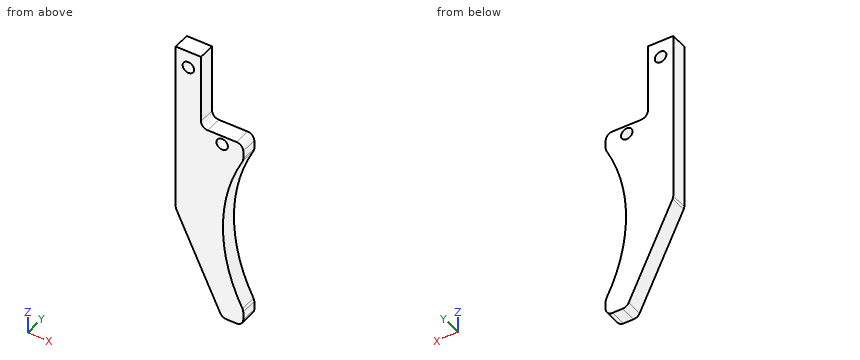
from build123d import *

# Parameters (mm, degrees)
BOSS_EXTRUDE1_DEPTH     = 6.35
CUT_EXTRUDE2_DEPTH      = 105.775
CUT_EXTRUDE2_DEPTH_BACK = 105.775
SKETCH5_R               = 2.159
FILLET1_R               = 2.54


with BuildPart() as part:
    # Sketch1 → Boss-Extrude1 (new body)
    with BuildSketch(Plane(origin=(0, 0, 0), x_dir=(1, 0, 0), z_dir=(0, 1, 0))):
        with BuildLine():
            Line((0, 0), (9.525, 0))
            Line((9.525, 0), (9.525, 28.48967645))
            Line((9.525, 28.48967645), (25.4, 28.48967645))
            Line((25.4, 28.48967645), (25.4, 34.83967645))
            ThreePointArc((25.4, 34.83967645), (17.756048931, 65.044838225), (25.4, 95.25))
            Line((25.4, 95.25), (25.4, 101.6))
            Line((25.4, 101.6), (17.4625, 101.6))
            Line((17.4625, 101.6), (0, 65.044838225))
            Line((0, 65.044838225), (0, 0))
        make_face()
    extrude(amount=BOSS_EXTRUDE1_DEPTH)

    # Sketch5 → Cut-Extrude2 (cut, two sides: drawn at the far end of the back side and taken through both)
    with BuildSketch(Plane(origin=(0, 3.175, 0), x_dir=(1, 0, 0), z_dir=(0, 1, 0)).offset(-CUT_EXTRUDE2_DEPTH_BACK)):
        with Locations(Location((17.4625, 31.75, 0), (0, 0, 270))):
            Circle(SKETCH5_R)
        with Locations(Location((4.7625, 6.35, 0), (0, 0, 270))):
            Circle(SKETCH5_R)
    extrude(amount=CUT_EXTRUDE2_DEPTH + CUT_EXTRUDE2_DEPTH_BACK, mode=Mode.SUBTRACT)

    # Fillet1
    fillet1_edges = [part.edges().sort_by_distance(p)[0] for p in [
        (0, 3.175, -65.044838225),
        (17.4625, 3.175, -101.6),
        (25.4, 3.175, -101.6),
        (25.4, 3.175, -95.25),
        (25.4, 3.175, -34.83967645),
        (25.4, 3.175, -28.48967645),
        (9.525, 3.175, -28.48967645),
    ]]
    fillet(fillet1_edges, radius=FILLET1_R)


solid = part.part
Model file for the job. Use its own axes, mm. Give positions to 0.01 mm unless a question says otherwise; leave off trailing zeros. Order: outer loops, then holes, each group sorted by start corner. A loop starts at its lowest first (then second) coordinate and runs counter-clockwise, first axis right, second up. Notation, with made-up numbers: (34, 12.5) - (89, 12.5) arc R29 cw to (89, 45.5) - close; hole circle Ø5 at (59.5, -18). An arc over 180 degrees is marked (long way). Return JSON: item names as keys, results as strings.
1) Cut at D-D, the plane z = -56. Give the cut face in (x, y), plus the area to 3 significant figures.
Geometry says:
{"outline": "(0, 0) - (18.4, 0) - (18.4, 6.35) - (0, 6.35) - close", "area": "117 mm²"}
2) Cut at B-B, the plane x = 21. Give the cut face in (y, z).
Geometry says:
{"outline": "(0, -101.6) - (6.35, -101.6) - (6.35, -85.08) - (0, -85.08) - close; (0, -45.01) - (6.35, -45.01) - (6.35, -28.49) - (0, -28.49) - close"}
3) Probe line 1 (X direction, y = 3, z = -31.75); line 2 (Z direction, x = 23, y = 1.25); line 3 (X direction, y = 4.75, z = -6.35) (1 decimal). List the from-to ranges inside material, lowest first. Write a range as from..to.
Geometry says:
{"line 1": "0..15.3, 19.62..25.4", "line 2": "-101.6..-90.31, -39.78..-28.49", "line 3": "0..2.6, 6.9..9.5"}
4) Flat gauge pins, fed straight in: P1, Ø2.5, axis at x = 17.46, z = -31.75, coming from the -Y side; P2, Ø2, axis at x = 21.5, y = 3, coming from the +Z side; P3, Ø3, axis at x = 9.5, y = 5, coming from the -Z side; P4, Ø1.9, axis at y = 4.5, z = -7, coming from the +X side (3 decimals). Where does each tip first touch, or does it go through?
Geometry says:
{"P1": "through", "P2": "z = -28.49", "P3": "z = -88.07", "P4": "x = 9.525"}
5) Cut at C-C, the plane y = 3. Count the separate pieces of the cut face and the enclosed holes in it, plus the area to 3 significant figures.
Geometry says:
{"separate pieces": "1", "enclosed holes": "2", "area": "1,470 mm²"}
